```python
from build123d import *

# Parameters (mm, degrees)
BOSS_EXTRUDE1_DEPTH = 12
BOSS_EXTRUDE2_DEPTH = 5.9
SKETCH3_R           = 1.7
CUT_EXTRUDE1_DEPTH  = 5.9
CUT_EXTRUDE2_DEPTH  = 3


with BuildPart() as part:
    # Sketch1 → Boss-Extrude1 (new body)
    with BuildSketch(Plane(origin=(0, 0, 0), x_dir=(1, 0, 0), z_dir=(0, 1, 0))):
        with BuildLine():
            Line((18.5, 75), (-18.5, 75))
            Line((-18.5, 75), (-15, -75))
            ThreePointArc((-15, -75), (0, -90), (15, -75))
            Line((15, -75), (18.5, 75))
        make_face()
    extrude(amount=BOSS_EXTRUDE1_DEPTH)

    # Sketch2 → Boss-Extrude2 (add)
    with BuildSketch(Plane.XZ):
        Polygon((-18.965, -95), (18.965, -95), (18.5, -75), (-18.5, -75), align=None)
        with BuildLine():
            Line((-18.5, -75), (18.5, -75))
            Line((18.5, -75), (15, 75))
            ThreePointArc((15, 75), (0, 90), (-15, 75))
            Line((-15, 75), (-18.5, -75))
        make_face()
    extrude(amount=-BOSS_EXTRUDE2_DEPTH)

    # Sketch3 → Cut-Extrude1 (cut)
    with BuildSketch(Plane.XZ):
        with Locations((-7.5, -85)):
            Circle(SKETCH3_R)
        with Locations((7.5, -85)):
            Circle(SKETCH3_R)
    extrude(amount=-CUT_EXTRUDE1_DEPTH, mode=Mode.SUBTRACT)

    # Sketch4 → Cut-Extrude2 (cut)
    with BuildSketch(Plane.XZ):
        Polygon((-7.5, -81.766838493), (-10.3, -83.383419246), (-10.3, -86.616580754), (-7.5, -88.233161507), (-4.7, -86.616580754), (-4.7, -83.383419246), align=None)
        Polygon((7.5, -81.766838493), (4.7, -83.383419246), (4.7, -86.616580754), (7.5, -88.233161507), (10.3, -86.616580754), (10.3, -83.383419246), align=None)
    extrude(amount=-CUT_EXTRUDE2_DEPTH, mode=Mode.SUBTRACT)


solid = part.part
```
Model file for the job. Use its own axes, mm. A direction names the side the tool comes from. Give positions to 0.01 mm unless a question says otherwise; leave off trailing zeros. Loops run counter-clockwise (first coordinate to the right, second up) from the corner with the lowest first, then second, coordinate; pieces in that order, holes last. Notation, with made-up numbers: (53, -12) -> (105, -12) arc R19 ccw to (105, 7) -> close; hole circle Ø1 at (35, 82.25). An arc over 180 degrees is marked (long way). Use CSV: the item, a comma, the result in double quotes. Start each with the question number.
1) Slice it at A-A on z = -85. Give the cut face in (x, y), plus the area to 3 significant figures.
2) Slice it at D-D on x = 0. Give the cut face in (y, z).
3) Slice it at B-B on x = -12. Give the cut face in (y, z).
4) Mould opens along X. For faces 4 (the cylindrical face through (0, 6, 90)), 5 (the flat face through (-8.8, 3, -86.4)), 6 (the flat face through (0, 3, -95)) say: released by +X, released by -X, zero draft, split by the parting line, or undercut.
5) Flat gauge pins, fed straight in: pin 1 Ø6 at (y, z) = (7, -24) entering from +X; pin 2 Ø6 at (y, z) = (1, -33) entering from +X; pin 3 Ø1 at (y, z) = (3, 4) entering from +X. Where does each tip first touch, or does it go through?
6) Wall check: line 1 (X direction, y = 3.65, z = -85); line 2 (Z direction, x = 10, y = 2.5); line 3 (Z direction, x = -6, y = 4). Give the ranges that are in metal, low to high.
7) Tool access for faces 1 (the flat face through (0, 9, -75)), 2 (the cylindrical face through (7.13, 4.43, -86.66)), 3 (the flat face through (10.3, 1, -85)): list every direction of +Z, -Z, +X, -X, +Y, -Y with a clear straight run to the whole face (end or side of a thin tool).
8) Slice it at C-C on z = -30. Give the cut face in (x, y).
Computed values:
1,outline,"(-18.73, 0) -> (-10.3, 0) -> (-10.3, 3) -> (-9.2, 3) -> (-9.2, 5.9) -> (-18.73, 5.9) -> close; (-5.8, 3) -> (-4.7, 3) -> (-4.7, 0) -> (4.7, 0) -> (4.7, 3) -> (5.8, 3) -> (5.8, 5.9) -> (-5.8, 5.9) -> close; (9.2, 3) -> (10.3, 3) -> (10.3, 0) -> (18.73, 0) -> (18.73, 5.9) -> (9.2, 5.9) -> close"
1,area,"168 mm^2"
2,outline,"(0, -95) -> (5.9, -95) -> (5.9, -75) -> (12, -75) -> (12, 90) -> (0, 90) -> close"
3,outline,"(0, -95) -> (5.9, -95) -> (5.9, -75) -> (12, -75) -> (12, 84) -> (0, 84) -> close"
4,face 4,"split by the parting line"
4,face 5,"undercut"
4,face 6,"zero draft"
5,pin 1,"stops at x = 17.38"
5,pin 2,"stops at x = 17.59"
5,pin 3,"stops at x = 16.67"
6,line 1,"x = -18.73 to -9.2, -5.8 to 5.8, 9.2 to 18.73"
6,line 2,"z = -95 to -86.79, -83.21 to 86.18"
6,line 3,"z = -95 to -85.8, -84.2 to 88.75"
7,face 1,"-Z, +X, -X, +Y"
7,face 2,"+Y, -Y"
7,face 3,"-Y"
8,outline,"(-17.45, 0) -> (17.45, 0) -> (17.45, 12) -> (-17.45, 12) -> close"
